from build123d import *

# Parameters (mm, degrees)
F0_W     = 24.5453510433
F0_H     = 19.5398386568
F1_DEPTH = 25.4
F2_SIZE  = 5.08
F3_R     = 3.6099939591
F4_DEPTH = 19.5408386568


with BuildPart() as f1:
    # F0 (on Front) → F1 (new body)
    with BuildSketch(Plane.XZ):
        with Locations((-12.2726755217, 9.7699193284)):
            Rectangle(F0_W, F0_H)
    extrude(amount=F1_DEPTH)

    # F2
    f2_edges = [f1.edges().sort_by_distance(p)[0] for p in [
        (-12.272676, 0, 0),
        (0, 0, 9.769919),
        (-12.272676, 0, 19.539839),
        (-24.545351, 0, 9.769919),
    ]]
    chamfer(f2_edges, length=F2_SIZE)

    # F3 (on face) → F4 (cut, through all)
    with BuildSketch(Plane.XY.offset(19.5398386568)):
        with Locations((-13.2677108049, -11.9031285867)):
            Circle(F3_R)
    extrude(amount=-F4_DEPTH, mode=Mode.SUBTRACT)


solid = f1.part
Build history of the part. All positions in model axes, mm. Coordinates: 2 decimals unless noted, no trailing zeros. Order: outer loops, then holes, each group sorted by start corner. A loop starts at its lowest first (then second) coordinate and runs counter-clockwise, first axis right, second up. Notation, with made-up numbers: (65, 23.25) - (98, 23.25) arc R18 cw to (98, 54.25) - close; hole circle Ø1 at (11, 87.5). An arc over 180 degrees is marked (long way). Write item = value, one per line. Start each with the question number.
1) Wall check: line 1 along Y through (x, z) = (-11.75, 4.5); line 2 along Y through (x, z) = (-12, 3.5); line 3 along X through (y, z) = (-10.5, 12.75). Give the ranges that are in metal, low to high. Write a range as from..to.
2) Saw through at B-B on x = -14.5. Write the cut outline in (y, z), then the cut area to 3 significant figures.
3) Saw through at C-C on z = 3. Write the cut outline in (x, y).
4) Saw through at A-A on y = -9.5. Write the cut outline in (x, z), then the cut area to 3 significant figures.
5) Two-plate mould, pull along Y, no slides. Class faces 1 (the face through (-9.824, -10.819, 9.907)), 2 (the face through (0, -15, 10)), 3 (the face through (-22.534, -3.069, 9.633)): pulls with the +Y half, pulls with the -Y half, needs draft (parallel to the pull), parting line crosses it, or undercut.
6) Saw through at D-D on x = -6.25. Write the cut outline in (y, z), then the cut area to 3 significant figures.
From the geometry:
q1.line_1 = -25.4..-15.18, -8.63..-0.58
q1.line_2 = -25.4..-15.28, -8.52..-1.58
q1.line_3 = -24.55..-16.59, -9.94..0
q2.outline = (-25.4, 0) - (-15.3, 0) - (-15.3, 19.54) - (-25.4, 19.54) - close; (-8.51, 0) - (-5.08, 0) - (0, 5.08) - (0, 14.46) - (-5.08, 19.54) - (-8.51, 19.54) - close
q2.area = 338 mm^2
q3.outline = (-24.55, -25.4) - (0, -25.4) - (0, -5.08) - (-3, -2.08) - (-21.55, -2.08) - (-24.55, -5.08) - close; hole circle Ø7.22 at (-13.27, -11.9)
q4.outline = (-24.55, 0) - (-15.96, 0) - (-15.96, 19.54) - (-24.55, 19.54) - close; (-10.57, 0) - (0, 0) - (0, 19.54) - (-10.57, 19.54) - close
q4.area = 374 mm^2
q5.face_1 = undercut
q5.face_2 = needs draft
q5.face_3 = pulls with the +Y half
q6.outline = (-25.4, 0) - (-5.08, 0) - (0, 5.08) - (0, 14.46) - (-5.08, 19.54) - (-25.4, 19.54) - close
q6.area = 471 mm^2
